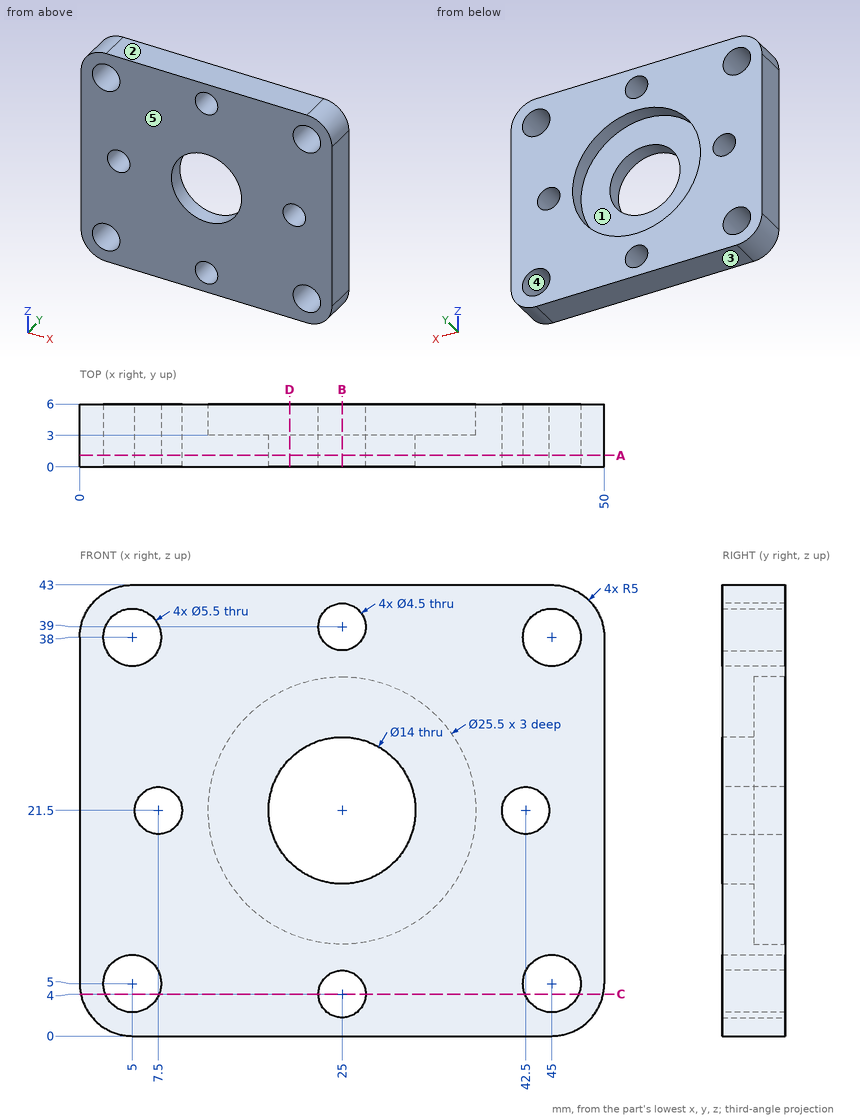
Design review of the part shown in the three views and the two pictorial views. Dimensions are in mm from the part's minimum x, y and z. A direction names the side the tool comes from. Give positions to 0.01 mm unless a question says otherwise; leave off trailing zeros. Order: outer loops, then holes, each group sorted by start corner. A loop starts at its lowest first (then second) coordinate and runs counter-clockwise, first axis right, second up. Notation, with made-up numbers: (41, -4) -> (70, -4) arc R29 ccw to (70, 21) -> close; hole circle Ø3 at (89, 39.5). An arc over 180 degrees is marked (long way). Write each question's results on one line, items separated by ' | '. Start each with the question number.
Q1. Add section B-B on x = 25. Give the boundary of the cut face in (y, z).
Q2. For pin 1 (5 mm diameter, centred on x = 5, z = 5, fed in from -Y); pin 2 (16 mm diameter, centred on x = 25, z = 21.5, fed in from +Y), all flat-tipped, find the tip position at first contact; note any pin that passes through.
Q3. Add section D-D on x = 20. Give the boundary of the cut face in (y, z), and give its area (3 significant figures).
Q4. Add section C-C on z = 4. Give the boundary of the cut face in (x, y), and give its area (3 significant figures).
Q5. Add section A-A on y = 1.1. State how many separate pieces and enclosed holes the cut face has, and give its area (3 significant figures).
Q6. Mouldability with a two-part tool opening along Z and no side actions: class the marked faces 3, 4 and 5 as +Z half, -Z half, draft (parallel to the pull), parting line (faces both ways), or undercut.
Q7. Wall thickness on L1, parallel to X at y = 4.25, z = 21.5; L2, parallel to X at y = 2.5, z = 39; L3, parallel to Z at x = 5.5, y = 5.3: over which ranges is each line inside the solid? List them lowest first. Write a range as from..to.
Q8. Machinability: for the marked faces 1 and 2, which of the approach directions +Z, -Z, +X, -X, +Y, -Y give a long, thin tool a straight path to every point of the face, cutting with its end or side? Answer none if there is none.
Found:
1) outline: (0, 0) -> (6, 0) -> (6, 1.75) -> (0, 1.75) -> close; (0, 6.25) -> (6, 6.25) -> (6, 8.75) -> (3, 8.75) -> (3, 14.5) -> (0, 14.5) -> close; (0, 28.5) -> (3, 28.5) -> (3, 34.25) -> (6, 34.25) -> (6, 36.75) -> (0, 36.75) -> close; (0, 41.25) -> (6, 41.25) -> (6, 43) -> (0, 43) -> close
2) pin 1: passes through | pin 2: stops at y = 3
3) outline: (0, 0) -> (6, 0) -> (6, 9.77) -> (3, 9.77) -> (3, 16.6) -> (0, 16.6) -> close; (0, 26.4) -> (3, 26.4) -> (3, 33.23) -> (6, 33.23) -> (6, 43) -> (0, 43) -> close | area: 158 mm2
4) outline: (0.1, 0) -> (2.44, 0) -> (2.44, 6) -> (0.1, 6) -> close; (7.56, 0) -> (22.75, 0) -> (22.75, 6) -> (7.56, 6) -> close; (27.25, 0) -> (42.44, 0) -> (42.44, 6) -> (27.25, 6) -> close; (47.56, 0) -> (49.9, 0) -> (49.9, 6) -> (47.56, 6) -> close | area: 210 mm2
5) separate pieces: 1 | enclosed holes: 9 | area: 1,820 mm2
6) face 3: -Z half | face 4: undercut | face 5: draft
7) L1: x = 0..5.25, 9.75..12.25, 37.75..40.25, 44.75..50 | L2: x = 0.1..2.44, 7.56..22.75, 27.25..42.44, 47.56..49.9 | L3: z = 0..2.3, 7.7..20.47, 22.53..35.3, 40.7..43
8) face 1: +Y | face 2: +Z, +X, -X, +Y, -Y
